The model under review builds one solid part; all positions refer to its coordinate system, in mm. Face numbers are marked on the shaded views. A direction names the side the tool comes from. Give positions to 0.01 mm unless a question says otherwise; leave off trailing zeros. Order: outer loops, then holes, each group sorted by start corner. A loop starts at its lowest first (then second) coordinate and runs counter-clockwise, first axis right, second up.
```python
from build123d import *

# Parameters (mm, degrees)
F1_DEPTH = 148


with BuildPart() as f1:
    # F0 (on Front) → F1 (new body)
    with BuildSketch(Plane.XZ):
        Polygon((145.814923, -11.975734), (145.814923, 148.024266), (135.014689, 70.738161), (135.014689, -11.975734), align=None)
        Polygon((-18.185077, 148.024266), (-18.185077, 130.001514), (135.014689, 130.001514), (135.014689, 70.738161), (145.814923, 148.024266), align=None)
    extrude(amount=-F1_DEPTH)


solid = f1.part
```
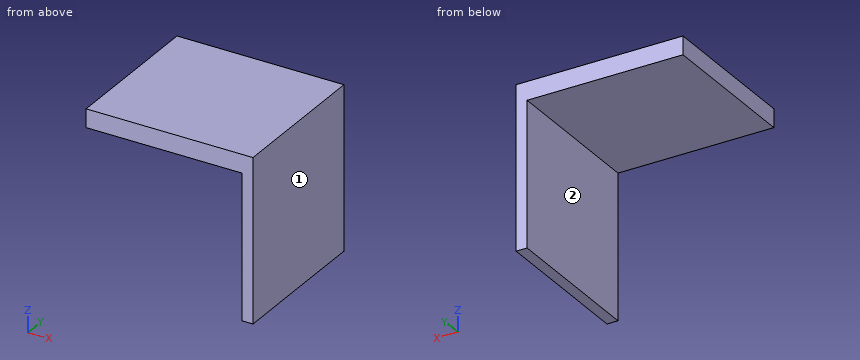
Item 1: Clearance check with flat-ended pins moving along their axes: pin 1 Ø6 at (y, z) = (30, 88) entering from -X; pin 2 Ø12 at (x, y) = (119.5, 36.5) entering from -Z. State where each tip first meets the part, or that it passes through.
Values found:
pin 1: stops at x = 135.01
pin 2: stops at z = 130
Item 2: Take a section at C-C (x = 2.5). Give the boundary of the cut face in (y, z).
Values found:
outline: (0, 130) - (148, 130) - (148, 148.02) - (0, 148.02) - close
Item 3: Take a section at A-A (y = 99.5). Give the boundary of the cut face in (x, z).
Values found:
outline: (-18.19, 130) - (135.01, 130) - (135.01, -11.98) - (145.81, -11.98) - (145.81, 148.02) - (-18.19, 148.02) - close
Item 4: For line 1 (X direction, y = 110, z = 56.5); line 2 (Z direction, x = -3, y = 83), list the stretches that pass through material, from the lowest coordinate up.
Values found:
line 1: x = 135.01 to 145.81
line 2: z = 130 to 148.02
Item 5: For the marked faces 1 and 2, list the 3-axis set-ups (+Z, -Z, +X, -X, +Y, -Y) from which the entire face can be reached by the end or side of a thin tool; tool diameter is ignored.
Values found:
face 1: +Z, -Z, +X, +Y, -Y
face 2: -Z, -X, +Y, -Y
Item 6: Take a section at B-B (z = 35). Give the boundary of the cut face in (x, y), and give its area (3 significant figures).
Values found:
outline: (135.01, 0) - (145.81, 0) - (145.81, 148) - (135.01, 148) - close
area: 1,600 mm2
